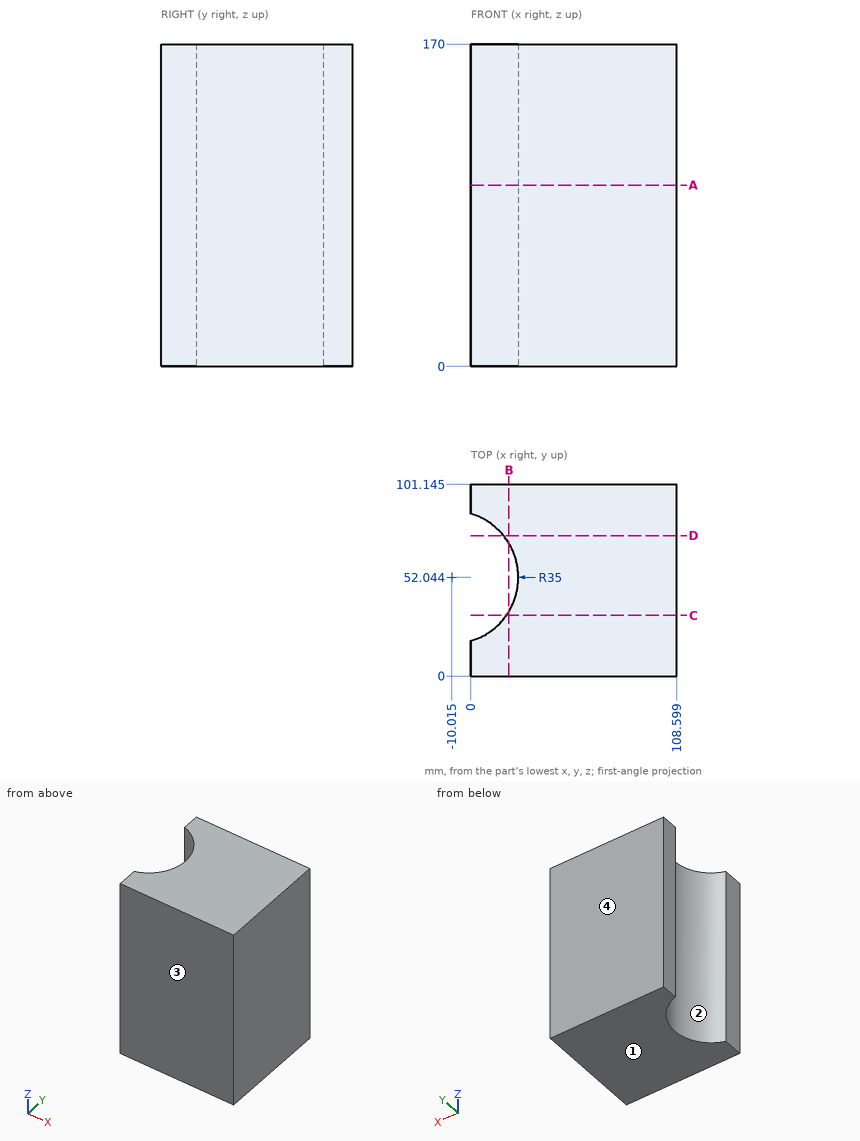
Geometry: see drawing. Coordinates: mm, zero at the bounding-box minimum. Coordinates: 2 decimals unless noted, no trailing zeros. Loops run counter-clockwise (first coordinate to the right, second up) from the corner with the lowest first, then second, coordinate; pieces in that order, holes last. Notation, with made-up numbers: (53, 77.25) - (99, 77.25) arc R24 ccw to (99, 109.25) - close; hole circle Ø2 at (12, 56). An arc over 180 degrees is marked (long way). Answer in a Markdown table with one row per item.
(1) Cut plane B-B on x = 20. Output: boundary loops of the cut face in (y, z) (1 decimal).
Model answer:
| item | result |
|---|---|
| outline | (0, 0) - (34, 0) - (34, 170) - (0, 170) - close; (70, 0) - (101.1, 0) - (101.1, 170) - (70, 170) - close |
(2) Material intervals for L1, parallel to Y at x = 14.5, z = 18.5 (1 decimal); L2, parallel to Y at x = 10.5, z = 114 (1 decimal); L3, parallel to X at y = 53.5, z = 125 (1 decimal), sorted ascending. Write a range as from..to.
Model answer:
| item | result |
|---|---|
| L1 | y = 0..27.1, 77..101.1 |
| L2 | y = 0..23.7, 80.4..101.1 |
| L3 | x = 25..108.6 |
(3) Mould query, pull axis Y, two halves, no side actions, for the marked faces 1, 2, 3 and 4. Classes: pulls with the +Y half, pulls with the -Y half, needs draft (parallel to the pull), parting line crosses it, or undercut.
Model answer:
| item | result |
|---|---|
| face 1 | needs draft |
| face 2 | undercut |
| face 3 | pulls with the -Y half |
| face 4 | pulls with the +Y half |
(4) Cut plane D-D on y = 74. Output: boundary loops of the cut face in (x, z), plus the area to 3 significant figures.
Model answer:
| item | result |
|---|---|
| outline | (17.24, 0) - (108.6, 0) - (108.6, 170) - (17.24, 170) - close |
| area | 15,500 mm² |
(5) Cut plane C-C on y = 32. Output: boundary loops of the cut face in (x, z).
Model answer:
| item | result |
|---|---|
| outline | (18.68, 0) - (108.6, 0) - (108.6, 170) - (18.68, 170) - close |
(6) Pin query (flat end, axial travel): P1, Ø4, axis at x = 14.5, z = 62, coming from the -Y side; P2, Ø10, axis at y = 64, z = 62.5, coming from the -X side; P3, Ø4, axis at y = 63.5, z = 65, coming from the -X side (1 decimal). Return the tip coordinate at first contact, or that it passes through.
Model answer:
| item | result |
|---|---|
| P1 | stops at y = 0 |
| P2 | stops at x = 20.6 |
| P3 | stops at x = 22.3 |
(7) Cut plane A-A on z = 95.5. Output: boundary loops of the cut face in (x, y) (1 decimal).
Model answer:
| item | result |
|---|---|
| outline | (0, 0) - (108.6, 0) - (108.6, 101.1) - (0, 101.1) - (0, 85.6) arc R35 cw to (0, 18.5) - close |
